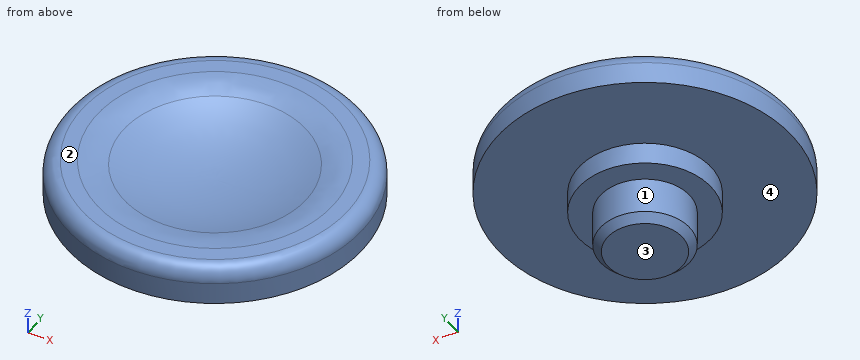
```python
from build123d import *

# Parameters (mm, degrees)
F2_R    = 5
F3_R    = 1
F4_SIZE = 0.5


with BuildPart() as f1:
    # F0 (on Front) → F1 (revolve)
    with BuildSketch(Plane.XZ):
        with BuildLine():
            Line((0, 5.45), (0, 0))
            Line((0, 0), (3.04, 0))
            Line((3.04, 0), (3.04, 2.95))
            Line((3.04, 2.95), (4.5, 2.95))
            Line((4.5, 2.95), (4.5, 4.45))
            Line((4.5, 4.45), (10, 4.45))
            Line((10, 4.45), (10, 6.95))
            Line((10, 6.95), (7, 6.95))
            ThreePointArc((7, 6.95), (3.579455, 5.829209), (0, 5.45))
        make_face()
    revolve(axis=Axis((0, 0, 3.81847), (0, 0, -1)))

    # F2
    f2_edges = [f1.edges().sort_by_distance(p)[0] for p in [
        (-7, 0, 6.95),
    ]]
    fillet(f2_edges, radius=F2_R)

    # F3
    f3_edges = [f1.edges().sort_by_distance(p)[0] for p in [
        (-10, 0, 6.95),
    ]]
    fillet(f3_edges, radius=F3_R)

    # F4
    f4_edges = [f1.edges().sort_by_distance(p)[0] for p in [
        (-3.04, 0, 0),
    ]]
    chamfer(f4_edges, length=F4_SIZE)


solid = f1.part
```
Design review of the part built by this model. Coordinates are the model's own, in mm. Face numbers are marked on the shaded views. A direction names the side the tool comes from. Give positions to 0.01 mm unless a question says otherwise; leave off trailing zeros. Loops run counter-clockwise (first coordinate to the right, second up) from the corner with the lowest first, then second, coordinate; pieces in that order, holes last. Notation, with made-up numbers: M 1.5,-21 L 35.5,-21 A15 cw 35.5,2 Z; hole C 80.25,-22.5 d11. An arc over 180 degrees is marked long. Return JSON: item names as keys, results as strings. Group by question number.
Item 1: Tool access review of the marked faces 3 and 4: name each direction out of +Z, -Z, +X, -X, +Y, -Y from which nothing blocks a thin tool from reaching the whole face with its end or side.
Item 2: Insertion check: pin 1 Ø2 at (x, z) = (-3, 3) entering from -Y; pin 2 Ø1 at (x, z) = (-3, 2) entering from -Y; pin 3 Ø1 at (x, z) = (-2, 5) entering from +Y; pin 4 Ø2.5 at (x, y) = (-0.5, -0.5) entering from -Z. Each pin has a flat end and moves straight along its axis. Give the tip position at first contact, or say it passes through.
Item 3: We need section A-A (z = 1.5). Give the boundary of the cut face in (x, y), and give its area (3 significant figures).
Item 4: For probe 1 along Z at (x, y) = (8.75, 0.75); probe 2 along Y at (x, z) = (1.5, 3.25), list the stretches that pass through material, from the lowest coordinate up.
Item 5: Mouldability with a two-part tool opening along Y and no side actions: class the marked faces 1 and 2 as released by +Y, released by -Y, zero draft, split by the parting line, or undercut.
Output:
{
 "1": {"face 3": "-Z, +X, -X, +Y, -Y", "face 4": "-Z"},
 "2": {"pin 1": "stops at y = -4.03", "pin 2": "stops at y = -1.73", "pin 3": "stops at y = 9.89", "pin 4": "stops at z = 0"},
 "3": {"outline": "C 0,0 d6.08", "area": "29.0 mm^2"},
 "4": {"probe 1": "z = 4.45 to 6.95", "probe 2": "y = -4.24 to 4.24"},
 "5": {"face 1": "split by the parting line", "face 2": "zero draft"}
}
